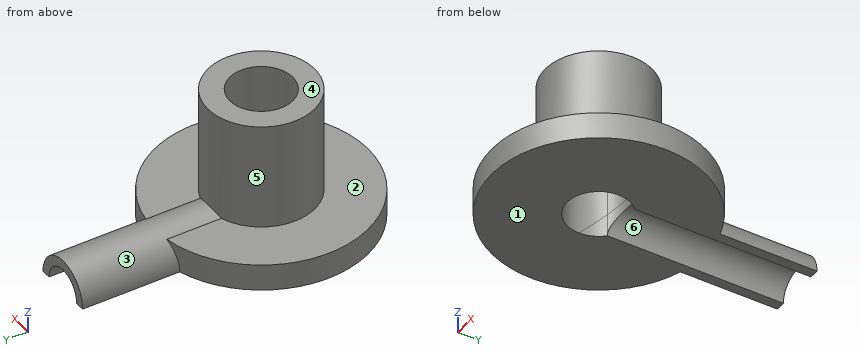
from build123d import *
from build123d.topology import SkipClean

# Parameters (mm, degrees)
SKETCH1_R           = 10
SKETCH1_R_2         = 2.95
BOSS_EXTRUDE1_DEPTH = 2.5
SKETCH2_R           = 5
SKETCH2_R_2         = 2.95
BOSS_EXTRUDE2_DEPTH = 10
SKETCH7_W           = 2.95
SKETCH7_H           = 18.687164731
REVOLVE7_ANGLE      = 180
SKETCH8_W           = 2.05
SKETCH8_H           = 18.687164731
SKETCH9_R           = 2.95
CUT_EXTRUDE1_DEPTH  = 5


with BuildPart() as part:
    # Sketch1 → Boss-Extrude1 (new body)
    with BuildSketch(Plane.XY):
        with Locations((102.341205301, 36.416113389)):
            Circle(SKETCH1_R)
        with Locations((102.341205301, 36.416113389)):
            Circle(SKETCH1_R_2, mode=Mode.SUBTRACT)
    extrude(amount=BOSS_EXTRUDE1_DEPTH)

    # Sketch2 → Boss-Extrude2 (add)
    with BuildSketch(Plane.XY.offset(2.5)):
        with Locations((102.341205301, 36.416113389)):
            Circle(SKETCH2_R)
        with Locations((102.341205301, 36.416113389)):
            Circle(SKETCH2_R_2, mode=Mode.SUBTRACT)
    extrude(amount=BOSS_EXTRUDE2_DEPTH)

    # Sketch7 → Revolve7 (revolve)
    with BuildSketch(Plane(origin=(0, 0, 0), x_dir=(-1, 0, 0), z_dir=(0, 0, -1))):
        with Locations((-103.816205301, 45.759695755)):
            Rectangle(SKETCH7_W, SKETCH7_H)
    revolve(axis=Axis((102.341205301, 36.416113389, 0), (0, -1, 0)), revolution_arc=REVOLVE7_ANGLE)

    # Sketch8 → Cut-Revolve2 (revolve, cut)
    with BuildSketch(Plane(origin=(0, 0, 0), x_dir=(-1, 0, 0), z_dir=(0, 0, -1))):
        with Locations((-103.366205301, 45.759695755)):
            Rectangle(SKETCH8_W, SKETCH8_H)
    revolve(axis=Axis((102.341205301, 36.416113389, 0), (0, 1, 0)), mode=Mode.SUBTRACT)

    # Sketch9 → Cut-Extrude1 (cut)
    with SkipClean():  # the faces are left unmerged after this step: merging them gives an invalid solid
        with BuildSketch(Plane(origin=(0, 0, 0), x_dir=(-1, 0, 0), z_dir=(0, 0, -1))):
            with Locations(Location((-102.341205301, 36.416113389, 0), (0, 0, 45.979535547))):
                Circle(SKETCH9_R)
        extrude(amount=-CUT_EXTRUDE1_DEPTH, mode=Mode.SUBTRACT)


solid = part.part
Input: part model. Units: mm. Frame: model coordinates. Face numbers are marked on the shaded views. A direction names the side the tool comes from. Coordinates: 2 decimals unless noted, no trailing zeros. Loops run counter-clockwise (first coordinate to the right, second up) from the corner with the lowest first, then second, coordinate; pieces in that order, holes last. Notation, with made-up numbers: (72.5, -26) -> (123.5, -26) arc R7 cw to (123.5, -17) -> close; hole circle Ø8 at (70, 37.5). An arc over 180 degrees is marked (long way). Write each question's results on one line, items separated by ' | '. Start each with the question number.
Q1. Section C-C, the plane x = 110. Return the cut outline in (y, z), plus the area to 3 significant figures.
Q2. Pull-direction query (X, two-part tool) for the marked faces 4, 5 and 6; classes: released by +X, released by -X, zero draft, split by the parting line, or undercut.
Q3. Pin query (flat end, axial travel): pin 1 (7 mm diameter, centred on x = 102.34, y = 36.42, fed in from -Z); pin 2 (1.5 mm diameter, centred on x = 101, y = 44.5, fed in from +Z); pin 3 (5 mm diameter, centred on y = 34, z = 8, fed in from +X); pin 4 (1.5 mm diameter, centred on y = 30.5, z = 2.5, fed in from -X). Return the tip coordinate at first contact, or that it passes through.
Q4. Section A-A, the plane y = 36.75. Return the cut outline in (x, z).
Q5. Section D-D, the plane y = 50.75. Return the cut outline in (x, z), plus the area to 3 significant figures.
Q6. Reachability of the marked faces 1, 2 and 3 from +Z, -Z, +X, -X, +Y, -Y: full face, straight path, thin tool, end or side. Return the list, or none.
Q7. Section B-B, the plane z = 8. Return the cut outline in (x, y).
Q8. Ray query, line 1 (Z direction, x = 111.25, y = 32.5); line 2 (X direction, y = 36, z = 1.5); line 3 (Y direction, x = 102.75, z = 4.75). Return the intervals inside material, ascending. Write a range as from..to.
Found:
1) outline: (29.99, 0) -> (42.85, 0) -> (42.85, 2.5) -> (29.99, 2.5) -> close | area: 32.1 mm2
2) face 4: zero draft | face 5: split by the parting line | face 6: undercut
3) pin 1: z = 0 | pin 2: z = 2.89 | pin 3: x = 107.34 | pin 4: x = 93.78
4) outline: (92.35, 0) -> (99.41, 0) -> (99.41, 12.5) -> (97.35, 12.5) -> (97.35, 2.5) -> (92.35, 2.5) -> close; (105.27, 0) -> (112.34, 0) -> (112.34, 2.5) -> (107.33, 2.5) -> (107.33, 12.5) -> (105.27, 12.5) -> close
5) outline: (99.39, 0) -> (100.29, 0) arc R2.05 cw to (104.39, 0) -> (105.29, 0) arc R2.95 ccw to start | area: 7.07 mm2
6) face 1: -Z, +X, -X, +Y, -Y | face 2: +Z | face 3: +Z, +Y
7) outline: circle Ø10 at (102.34, 36.42); hole circle Ø5.9 at (102.34, 36.42)
8) line 1: 0..2.5 | line 2: 92.35..99.42, 105.26..112.33 | line 3: 31.43..33.49, 39.34..41.4
